Part model, mm, in its own coordinate system. Face numbers are marked on the shaded views. A direction names the side the tool comes from. Coordinates: 2 decimals unless noted, no trailing zeros. Order: outer loops, then holes, each group sorted by start corner. A loop starts at its lowest first (then second) coordinate and runs counter-clockwise, first axis right, second up.
1) Tool access for the marked faces 1 and 2: list every direction of +Z, -Z, +X, -X, +Y, -Y with a clear straight run to the whole face (end or side of a thin tool).
2) Pin check, flat tips, straight feed: pin 1 Ø2.5 at (x, z) = (-33.34, 0) entering from -Y; pin 2 Ø1 at (x, y) = (1, -7) entering from +Z; pin 3 Ø1.5 at (x, y) = (-13, -5.5) entering from -Z. Stop position of each tip, or through.
3) Wall check: L1, parallel to Y at x = -30, z = -8 (3 decimals); L2, parallel to X at y = -17, z = 2.5; L3, parallel to Z at x = 14.5, y = -3.25. Give the ranges that are in metal, low to high.
4) Cut at A-A (y = 1). Give the number of separate pieces and of enclosed holes in the cut face, and give its area (3 significant figures).
5) Cut at D-D (z = 30.5). List the corners of the cut face in (x, y) (3 decimals), and give its area (3 significant figures).
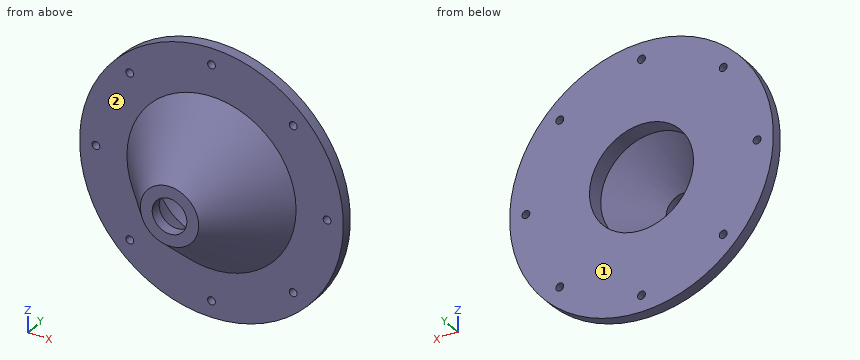
```python
from build123d import *

# Parameters (mm, degrees)
SKETCH1_R                 = 38.04031
BOSS_EXTRUDE1_DEPTH       = 3.175
TAP_DRILL_FOR_4_40_TAP1_D = 2.2606
CIRPATTERN1_COUNT         = 8
SKETCH5_R                 = 25.4
BOSS_EXTRUDE2_DEPTH       = 19.05
CUT_EXTRUDE1_DEPTH        = 59.207224593
CUT_EXTRUDE1_DEPTH_BACK   = 59.207224593
SKETCH6_R                 = 5
SKETCH7_R                 = 15
CUT_EXTRUDE2_DEPTH        = 5.08


with BuildPart() as part:
    # Sketch1 → Boss-Extrude1 (new body)
    with BuildSketch(Plane(origin=(0, 0, 0), x_dir=(1, 0, 0), z_dir=(0, 1, 0))):
        with Locations(Location((0, 0, 0), (0, 0, 270))):
            Circle(SKETCH1_R)
    extrude(amount=BOSS_EXTRUDE1_DEPTH)

    # Tap Drill for #4-40 Tap1 (through all)
    with Locations(Plane(origin=(0, 0, 0), x_dir=(-1, 0, 0), z_dir=(0, -1, 0))):
        with Locations((0, -33.3375)):
            tap_drill_for_4_40_tap1 = Hole(TAP_DRILL_FOR_4_40_TAP1_D / 2)

    # CirPattern1: Tap Drill for #4-40 Tap1 ×8 about axis
    cirpattern1_axis = Axis((0, 0, 0), (0, 1, 0))
    for i in range(1, CIRPATTERN1_COUNT):
        add(tap_drill_for_4_40_tap1.rotate(cirpattern1_axis, i * 360 / CIRPATTERN1_COUNT), mode=Mode.SUBTRACT)

    # Sketch5 → Boss-Extrude2 (add)
    with BuildSketch(Plane.XZ):
        with Locations(Location((0, 0, 0), (0, 0, 90))):
            Circle(SKETCH5_R)
    extrude(amount=BOSS_EXTRUDE2_DEPTH)

    # Sketch6 → Cut-Extrude1 (cut, two sides: drawn at the far end of the back side and taken through both)
    with BuildSketch(Plane.XZ.offset(19.05).offset(-CUT_EXTRUDE1_DEPTH_BACK)):
        with Locations(Location((0, 0, 0), (0, 0, 270))):
            Circle(SKETCH6_R)
    extrude(amount=CUT_EXTRUDE1_DEPTH + CUT_EXTRUDE1_DEPTH_BACK, mode=Mode.SUBTRACT)

    # Sketch7 → Cut-Extrude2 (cut)
    with BuildSketch(Plane(origin=(0, 3.175, 0), x_dir=(1, 0, 0), z_dir=(0, 1, 0))):
        with Locations(Location((0, 0, 0), (0, 0, 270))):
            Circle(SKETCH7_R)
    extrude(amount=-CUT_EXTRUDE2_DEPTH, mode=Mode.SUBTRACT)

    # Cut-Loft1: read off the stored shape, not the designer's step
    # Cut-Loft1: loft between two sections, ruled curve by curve
    cut_loft1_from = [
        Edge.make_bspline([(0, -1.905, 15), (-30, -1.905, 15), (-30, -1.905, -15), (0, -1.905, -15), (30, -1.905, -15), (30, -1.905, 15), (0, -1.905, 15)], [0, 0, 0, 0, 0.5, 0.5, 0.5, 1, 1, 1, 1], 3, [1, 0.333333333, 0.333333333, 1, 0.333333333, 0.333333333, 1]),
    ]
    cut_loft1_to = [
        Edge.make_bspline([(-1.365853626, -15.875, 4.809827842), (-10.985509311, -15.875, 2.07812059), (-8.253802058, -15.875, -7.541535095), (1.365853626, -15.875, -4.809827842), (10.985509311, -15.875, -2.07812059), (8.253802058, -15.875, 7.541535095), (-1.365853626, -15.875, 4.809827842)], [0, 0, 0, 0, 0.5, 0.5, 0.5, 1, 1, 1, 1], 3, [1, 0.333333333, 0.333333333, 1, 0.333333333, 0.333333333, 1]),
    ]
    cut_loft1 = Solid(Shell([*[Face.make_surface_from_curves(cut_loft1_from[k], cut_loft1_to[k]) for k in range(1)], Face(Wire(cut_loft1_from)), Face(Wire(cut_loft1_to))]))
    add(cut_loft1, mode=Mode.SUBTRACT)

    # Sketch10 → Cut-Revolve1 (revolve, cut)
    with BuildSketch(Plane.XY):
        Polygon((-25.4, 0), (-24.4, 0), (-8.415152026, -19.05), (-25.4, -19.05), align=None)
    revolve(axis=Axis((0, 0, 0), (0, -1, 0)), mode=Mode.SUBTRACT)


solid = part.part
```
Geometry check:
1. face 1: +Z, -Z, +X, -X, +Y
1. face 2: -Y
2. pin 1: stops at y = 0
2. pin 2: stops at z = 18.92
2. pin 3: stops at z = -15.94
3. L1: y = 0 to 3.175
3. L2: x = -9.82 to -4.33, 4.33 to 9.82
3. L3: z = -16.11 to 16.11
4. separate pieces: 1
4. enclosed holes: 9
4. area: 3,810 mm2
5. outline: (-22.734, 0) - (22.734, 0) - (22.734, 3.175) - (-22.734, 3.175) - close
5. area: 144 mm2
